from build123d import *

# Parameters (mm, degrees)
SKETCH1_W           = 101.6
SKETCH1_H           = 50.8
BOSS_EXTRUDE1_DEPTH = 25.4
SKETCH2_R           = 5.842
BOSS_EXTRUDE2_DEPTH = 25.4


with BuildPart() as part:
    # Sketch1 → Boss-Extrude1 (new body)
    with BuildSketch(Plane(origin=(0, 0, 0), x_dir=(1, 0, 0), z_dir=(0, 1, 0))):
        Rectangle(SKETCH1_W, SKETCH1_H)
    extrude(amount=BOSS_EXTRUDE1_DEPTH)

    # Sketch2 → Boss-Extrude2 (add)
    with BuildSketch(Plane.XY.offset(25.4)):
        with Locations(Location((0, 12.7, 0), (0, 0, 180))):
            Circle(SKETCH2_R)
    boss_extrude2 = extrude(amount=BOSS_EXTRUDE2_DEPTH)

    # Mirror1: Boss-Extrude2 across plane
    add(boss_extrude2.mirror(Plane.XY))


solid = part.part
Source: CAD feature listing. Evaluate the final solid. Frame: model axes, mm. A direction names the side the tool comes from. Round coordinates to 2 decimals unless told otherwise and drop trailing zeros. Order: outer loops, then holes, each group sorted by start corner. A loop starts at its lowest first (then second) coordinate and runs counter-clockwise, first axis right, second up. Notation, with made-up numbers: (19, 20) -> (46, 20) arc R26 cw to (46, 45) -> close; hole circle Ø10 at (10.25, -25). An arc over 180 degrees is marked (long way). Answer as CSV lines item,"result".
Item 1: Line query: L1, parallel to Z at x = 18.5, y = 4; L2, parallel to Y at x = 4.5, z = 32; L3, parallel to X at y = 14.5, z = 27.5. Output: solid intervals per line, ascending.
A:
L1,"-25.4 to 25.4"
L2,"8.97 to 16.43"
L3,"-5.56 to 5.56"
Item 2: Section C-C, the plane x = -28. Return loops of the section in (y, z), plus the area to 3 significant figures.
A:
outline,"(0, -25.4) -> (25.4, -25.4) -> (25.4, 25.4) -> (0, 25.4) -> close"
area,"1,290 mm²"
Item 3: Section A-A, the plane y = 12.7. Return loops of the section in (x, z), plus the area to 3 significant figures.
A:
outline,"(-50.8, -25.4) -> (-5.84, -25.4) -> (-5.84, -50.8) -> (5.84, -50.8) -> (5.84, -25.4) -> (50.8, -25.4) -> (50.8, 25.4) -> (5.84, 25.4) -> (5.84, 50.8) -> (-5.84, 50.8) -> (-5.84, 25.4) -> (-50.8, 25.4) -> close"
area,"5,750 mm²"
Item 4: Pin query (flat end, axial travel): pin 1 Ø5 at (y, z) = (4, 33) entering from -X; pin 2 Ø1.5 at (x, y) = (-22.5, 6.5) entering from -Z; pin 3 Ø4 at (x, y) = (37, 11.5) entering from +Z; pin 4 Ø3 at (y, z) = (11.5, 40.5) entering from -X. Return the tip coordinate at first contact, or that it passes through.
A:
pin 1,"through"
pin 2,"z = -25.4"
pin 3,"z = 25.4"
pin 4,"x = -5.84"
Item 5: Reachability of faces 1 (the face through (0, 13, 50.8)), 2 (the face through (1.266, 18.403, 37.922)), 3 (the face through (1.266, 18.403, -37.922)) from +Z, -Z, +X, -X, +Y, -Y: full face, straight path, thin tool, end or side. Return the list, or none.
A:
face 1,"+Z, +X, -X, +Y, -Y"
face 2,"+Z"
face 3,"-Z"
Item 6: Section B-B, the plane x = 0. Return loops of the section in (y, z).
A:
outline,"(0, -25.4) -> (6.86, -25.4) -> (6.86, -50.8) -> (18.54, -50.8) -> (18.54, -25.4) -> (25.4, -25.4) -> (25.4, 25.4) -> (18.54, 25.4) -> (18.54, 50.8) -> (6.86, 50.8) -> (6.86, 25.4) -> (0, 25.4) -> close"
Item 7: Section D-D, the plane y = 21.25. Return loops of the section in (x, z).
A:
outline,"(-50.8, -25.4) -> (50.8, -25.4) -> (50.8, 25.4) -> (-50.8, 25.4) -> close"
